Job drawing, mm, ordinate dimensions from the low corner. One solid piece. Give positions to 0.01 mm unless a question says otherwise; leave off trailing zeros. Write each loop counter-clockwise with the first axis right and the second up, starting at its lowest first coordinate (ties: lowest second). Pieces come first, ordered by that corner, then holes. Notation, with made-up numbers: (7.25, -26) - (13.25, -26) arc R19 cw to (13.25, -8) - close; hole circle Ø10 at (4.5, -24). An arc over 180 degrees is marked (long way). Answer as a JSON object with one key per item and string values.
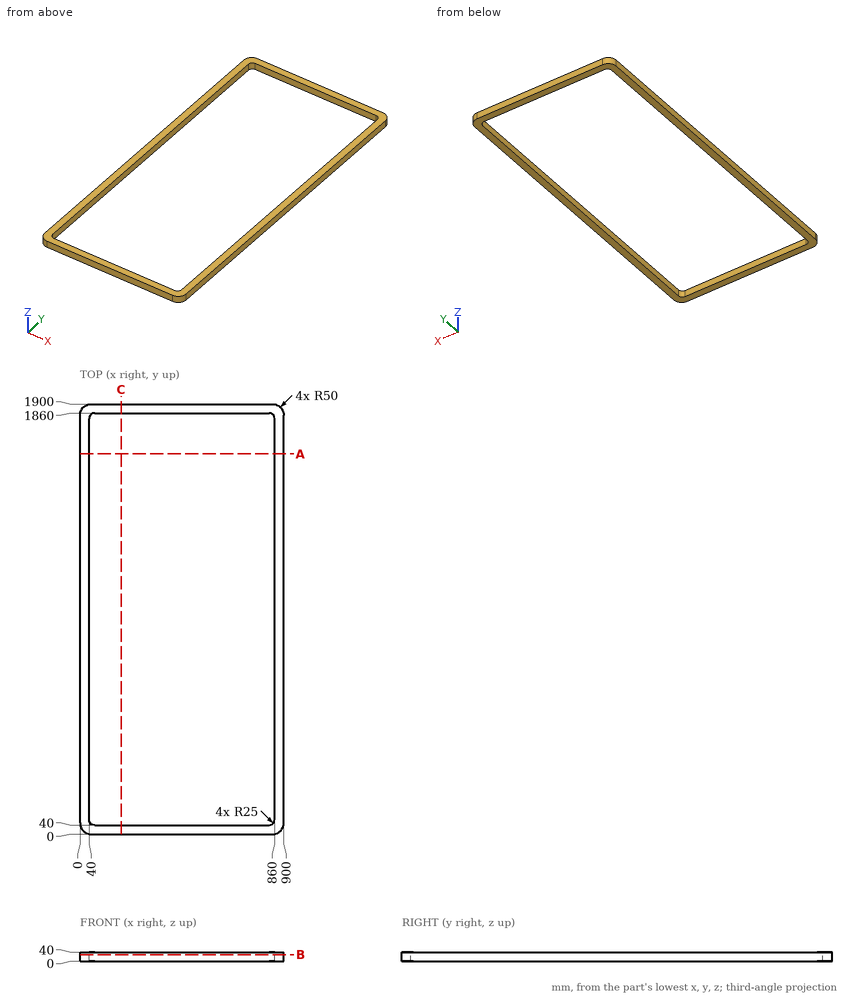
Item 1: Cut at A-A (y = 1680). Give the cut face in (x, z).
Entries:
{"outline": "(0, 0) - (40, 0) - (40, 40) - (0, 40) - close; (860, 0) - (900, 0) - (900, 40) - (860, 40) - close"}
Item 2: Cut at C-C (x = 182). Give the cut face in (y, z), and give its area (3 significant figures).
Entries:
{"outline": "(0, 0) - (40, 0) - (40, 40) - (0, 40) - close; (1860, 0) - (1900, 0) - (1900, 40) - (1860, 40) - close", "area": "3,200 mm2"}
Item 3: Cut at B-B (z = 29.5). Give the cut face in (x, y).
Entries:
{"outline": "(0, 50) arc R50 ccw to (50, 0) - (850, 0) arc R50 ccw to (900, 50) - (900, 1850) arc R50 ccw to (850, 1900) - (50, 1900) arc R50 ccw to (0, 1850) - close; hole (40, 65) arc R25 ccw to (65, 40) - (835, 40) arc R25 ccw to (860, 65) - (860, 1835) arc R25 ccw to (835, 1860) - (65, 1860) arc R25 ccw to (40, 1835) - close"}
Item 4: Probe line 1 (X direction, y = 788.5, z = 35); line 2 (Y direction, x = 657, z = 13). List the from-to ranges inside material, lowest first. Write a range as from..to.
Entries:
{"line 1": "0..40, 860..900", "line 2": "0..40, 1860..1900"}
